from build123d import *

# Parameters (mm, degrees)
F0_W     = 31.75
F0_H     = 12.7
F1_DEPTH = 63.5
F3_DEPTH = 25.401
F2_R     = 9.525
F4_DEPTH = 25.401


with BuildPart() as f1:
    # F0 (on Front) → F1 (new body)
    with BuildSketch(Plane.XZ):
        Polygon((0, 12.7), (0, 0), (63.5, 0), (63.5, 12.7), (47.625, 12.7), (15.875, 12.7), align=None)
        with Locations((31.75, 19.05)):
            Rectangle(F0_W, F0_H)
    extrude(amount=F1_DEPTH)

    # F2 (on face) → F3 (cut, through all)
    with BuildSketch(Plane(origin=(0, 0, 0), x_dir=(1, 0, 0), z_dir=(0, 0, -1))):
        with BuildLine():
            ThreePointArc((0, 31.75), (9.2993596973, 54.2006403027), (31.75, 63.5))
            Line((31.75, 63.5), (0, 63.5))
            Line((0, 63.5), (0, 31.75))
        make_face()
        with BuildLine():
            ThreePointArc((31.75, 63.5), (54.2006403027, 54.2006403027), (63.5, 31.75))
            Line((63.5, 31.75), (63.5, 63.5))
            Line((63.5, 63.5), (31.75, 63.5))
        make_face()
        with BuildLine():
            Line((0, 0), (31.75, 0))
            ThreePointArc((31.75, 0), (9.2993596973, 9.2993596973), (0, 31.75))
            Line((0, 31.75), (0, 0))
        make_face()
        with BuildLine():
            Line((63.5, 0), (63.5, 31.75))
            ThreePointArc((63.5, 31.75), (54.2006403027, 9.2993596973), (31.75, 0))
            Line((31.75, 0), (63.5, 0))
        make_face()
    extrude(amount=-F3_DEPTH, mode=Mode.SUBTRACT)

    # F2 (on face) → F4 (cut, through all)
    with BuildSketch(Plane(origin=(0, 0, 0), x_dir=(1, 0, 0), z_dir=(0, 0, -1))):
        with BuildLine():
            ThreePointArc((28.5812072396, 56.9515625), (31.75, 57.15), (34.9187927604, 56.9515625))
            ThreePointArc((34.9187927604, 56.9515625), (34.9234478107, 57.0507327204), (34.925, 57.15))
            ThreePointArc((34.925, 57.15), (31.6507327204, 60.3234478107), (28.5812072396, 56.9515625))
        make_face()
        with BuildLine():
            ThreePointArc((28.5812072396, 56.9515625), (31.75, 53.975), (34.9187927604, 56.9515625))
            ThreePointArc((34.9187927604, 56.9515625), (31.75, 57.15), (28.5812072396, 56.9515625))
        make_face()
        with BuildLine():
            ThreePointArc((9.525, 31.75), (8.6641590333, 33.9237739001), (6.5484375, 34.9187927604))
            ThreePointArc((6.5484375, 34.9187927604), (6.35, 31.75), (6.5484375, 28.5812072396))
            ThreePointArc((6.5484375, 28.5812072396), (8.6641590333, 29.5762260999), (9.525, 31.75))
        make_face()
        with BuildLine():
            ThreePointArc((6.5484375, 28.5812072396), (6.35, 31.75), (6.5484375, 34.9187927604))
            ThreePointArc((6.5484375, 34.9187927604), (3.175, 31.75), (6.5484375, 28.5812072396))
        make_face()
        with BuildLine():
            ThreePointArc((34.925, 6.35), (34.9234478107, 6.4492672796), (34.9187927604, 6.5484375))
            ThreePointArc((34.9187927604, 6.5484375), (31.75, 6.35), (28.5812072396, 6.5484375))
            ThreePointArc((28.5812072396, 6.5484375), (31.6507327204, 3.1765521893), (34.925, 6.35))
        make_face()
        with BuildLine():
            ThreePointArc((28.5812072396, 6.5484375), (31.75, 6.35), (34.9187927604, 6.5484375))
            ThreePointArc((34.9187927604, 6.5484375), (31.75, 9.525), (28.5812072396, 6.5484375))
        make_face()
        with BuildLine():
            ThreePointArc((56.9515625, 34.9187927604), (57.1003420835, 33.3375), (57.15, 31.75))
            ThreePointArc((57.15, 31.75), (57.1003420835, 30.1625), (56.9515625, 28.5812072396))
            ThreePointArc((56.9515625, 28.5812072396), (59.3237739001, 29.4358409667), (60.325, 31.75))
            ThreePointArc((60.325, 31.75), (59.3237739001, 34.0641590333), (56.9515625, 34.9187927604))
        make_face()
        with BuildLine():
            ThreePointArc((56.9515625, 28.5812072396), (57.1003420835, 30.1625), (57.15, 31.75))
            ThreePointArc((57.15, 31.75), (57.1003420835, 33.3375), (56.9515625, 34.9187927604))
            ThreePointArc((56.9515625, 34.9187927604), (53.975, 31.75), (56.9515625, 28.5812072396))
        make_face()
        with Locations((31.75, 31.75)):
            Circle(F2_R)
    extrude(amount=-F4_DEPTH, mode=Mode.SUBTRACT)


solid = f1.part
Geometry: final body of the model. Coordinates: model frame, mm. A direction names the side the tool comes from. Give positions to 0.01 mm unless a question says otherwise; leave off trailing zeros. Write each loop counter-clockwise with the first axis right and the second up, starting at its lowest first coordinate (ties: lowest second). Pieces come first, ordered by that corner, then holes.
(1) Cut plane B-B, the plane x = 37.5. Return loops of the section in (y, z).
(2) Ray query, line 1 (Y direction, x = 31.75, z = 9.5) (3 decimals); line 2 (X direction, y = -31.75, z = 6) (3 decimals); line 3 (X direction, y = -31.75, z = 18) (3 decimals). Return the intervals inside material, ascending.
(3) Mould query, pull axis X, two halves, no side actions, for faces 3 (the cylindrical face through (29.69, -22.45, 12.52)), 4 (the flat face through (52, -31, 12.7)), 5 (the flat face through (47.625, -31, 19)). Classes: released by +X, released by -X, zero draft, split by the parting line, or undercut.
(4) Cut plane C-C, the plane z = 5.25. Return loops of the section in (x, y) (3 decimals), then the cut area to 3 significant figures.
(5) Access query for faces 1 (the flat face through (15.875, -31, 19)), 2 (the flat face through (38, -24, 0)). Directions: +Z, -Z, +X, -X, +Y, -Y. A direction counts if a zero-diameter tool reaches every point of the face in a straight line with its end or side. Return the directions, or none.
(6) Cut plane A-A, the plane z = 19. Return loops of the section in (x, y) (3 decimals), then the cut area to 3 significant figures.
(7) Cut plane D-D, the plane x = 30.5. Return loops of the section in (y, z).
(8) First-contact query: P1, Ø14, axis at y = -45.5, z = 17.5, coming from the +X side; P2, Ø10, axis at x = 53, y = -51.5, coming from the +Z side; P3, Ø2, axis at x = 9, y = -21, coming from the -Z side; P4, Ø1, axis at y = -42, z = 16, coming from the -X side (3 decimals). Flat tips, straight axial feed; report the tip coordinate or a pass-through.
Values follow:
1. outline: (-62.97, 0) - (-39.34, 0) - (-39.34, 25.4) - (-62.97, 25.4) - close; (-24.16, 0) - (-0.53, 0) - (-0.53, 25.4) - (-24.16, 25.4) - close
2. line 1: y = -63.5 to -60.325, -53.975 to -41.275, -22.225 to -9.525, -3.175 to 0
2. line 2: x = 0 to 3.175, 9.525 to 22.225, 41.275 to 53.975, 60.325 to 63.5
2. line 3: x = 15.875 to 22.225, 41.275 to 47.625
3. face 3: undercut
3. face 4: zero draft
3. face 5: released by +X
4. outline: circle Ø63.5 at (31.75, -31.75); hole circle Ø6.35 at (6.35, -31.75); hole circle Ø19.05 at (31.75, -31.75); hole circle Ø6.35 at (31.75, -57.15); hole circle Ø6.35 at (31.75, -6.35); hole circle Ø6.35 at (57.15, -31.75)
4. area: 2,760 mm2
5. face 1: +Z, -X, +Y, -Y
5. face 2: -Z, +X, -X, +Y, -Y
6. outline: (15.875, -59.246) arc R31.75 ccw to (47.625, -59.246) - (47.625, -4.254) arc R31.75 ccw to (15.875, -4.254) - close; hole circle Ø19.05 at (31.75, -31.75); hole circle Ø6.35 at (31.75, -57.15); hole circle Ø6.35 at (31.75, -6.35)
6. area: 1,580 mm2
7. outline: (-63.48, 0) - (-60.07, 0) - (-60.07, 25.4) - (-63.48, 25.4) - close; (-54.23, 0) - (-41.19, 0) - (-41.19, 25.4) - (-54.23, 25.4) - close; (-22.31, 0) - (-9.27, 0) - (-9.27, 25.4) - (-22.31, 25.4) - close; (-3.43, 0) - (-0.02, 0) - (-0.02, 25.4) - (-3.43, 25.4) - close
8. P1: stops at x = 62.3
8. P2: stops at z = 12.7
8. P3: stops at z = 0
8. P4: stops at x = 15.875
